Can you work these out from the model? Positions are in its coordinate system, mm. A direction names the side the tool comes from. Coordinates: 2 decimals unless noted, no trailing zeros. Order: outer loops, then holes, each group sorted by start corner. A loop starts at its lowest first (then second) coordinate and runs counter-clockwise, first axis right, second up. Notation, with made-up numbers: M 70.5,25 L 87.5,25 A31 ccw 87.5,49 Z; hole C 84.25,-21.5 d6. An arc over 180 degrees is marked long. Answer as a JSON object with one key per item and string values.
Autodesk Fusion 360 part; units mm, degrees
sketch "Sketch1" plane through (0, 0, 0) normal (1, 0, 0) x (0, 0, -1)
  circle A0 centre (-17.75, 2.25) radius 1.25
  circle A1 centre (-2.25, 2.25) radius 1.25
  circle A2 centre (-17.75, 17.75) radius 1.25
  circle A3 centre (-2.25, 17.75) radius 1.25
  circle A4 centre (-10, 10) radius 2.7
  line L0 (-13.1, 0) -> (-13.1, 1.7)
  line L1 (-13.1, 1.7) -> (-15.5, 1.7)
  line L2 (-15.5, 1.7) -> (-15.5, 3.2272)
  line L3 (-13.1, 0) -> (-20, 0)
  line L4 (-13.1, 0) -> (-6.9, 0) construction
  line L5 (-10, 15.8164) -> (-10, 4.0346) construction
  line L6 (-15.4081, 10) -> (-4.6511, 10) construction
  line L7 (-16.7728, 4.5) -> (-18.3, 4.5)
  line L8 (-18.3, 4.5) -> (-18.3, 6.9)
  line L9 (-18.3, 6.9) -> (-20, 6.9)
  line L10 (-20, 6.9) -> (-20, 0)
  line L11 (0, 6.9) -> (0, 0)
  line L12 (-1.7, 6.9) -> (0, 6.9)
  line L13 (-1.7, 4.5) -> (-1.7, 6.9)
  line L14 (-3.2272, 4.5) -> (-1.7, 4.5)
  line L15 (-4.5, 1.7) -> (-4.5, 3.2272)
  line L16 (-6.9, 1.7) -> (-4.5, 1.7)
  line L17 (-6.9, 0) -> (-6.9, 1.7)
  line L18 (-6.9, 0) -> (0, 0)
  line L19 (-6.9, 20) -> (-6.9, 18.3)
  line L20 (-6.9, 18.3) -> (-4.5, 18.3)
  line L21 (-4.5, 18.3) -> (-4.5, 16.7728)
  line L22 (-3.2272, 15.5) -> (-1.7, 15.5)
  line L23 (-1.7, 15.5) -> (-1.7, 13.1)
  line L24 (-1.7, 13.1) -> (0, 13.1)
  line L25 (0, 13.1) -> (0, 20)
  line L26 (-6.9, 20) -> (0, 20)
  line L27 (-13.1, 20) -> (-13.1, 18.3)
  line L28 (-13.1, 20) -> (-20, 20)
  line L29 (-13.1, 18.3) -> (-15.5, 18.3)
  line L30 (-15.5, 18.3) -> (-15.5, 16.7728)
  line L31 (-16.7728, 15.5) -> (-18.3, 15.5)
  line L32 (-18.3, 15.5) -> (-18.3, 13.1)
  line L33 (-18.3, 13.1) -> (-20, 13.1)
  line L34 (-20, 13.1) -> (-20, 20)
  line L35 (-16.7728, 4.5) -> (-13.8, 7.4728)
  line L36 (-7.4728, 13.8) -> (-4.5, 16.7728)
  line L37 (-15.5, 16.7728) -> (-12.5272, 13.8)
  line L38 (-6.2, 7.4728) -> (-3.2272, 4.5)
  line L39 (-15.5, 3.2272) -> (-12.5272, 6.2)
  line L40 (-6.2, 12.5272) -> (-3.2272, 15.5)
  line L41 (-16.7728, 15.5) -> (-13.8, 12.5272)
  line L42 (-7.4728, 6.2) -> (-4.5, 3.2272)
  line L43 (-12.5272, 13.8) -> (-7.4728, 13.8)
  line L44 (-6.2, 12.5272) -> (-6.2, 7.4728)
  line L45 (-7.4728, 6.2) -> (-12.5272, 6.2)
  line L46 (-13.8, 7.4728) -> (-13.8, 12.5272)
  line L47 (-17.75, 17.75) -> (-2.25, 2.25) construction
  line L48 (-17.75, 2.25) -> (-2.25, 17.75) construction
  dimension "d3" = 2.5
  dimension "d13" = 15.5
  dimension "d14" = 5.4
  dimension "d16" = 2.4
  dimension "d19" = 1.7
  dimension "d21" = 3.1
  dimension "d29" = 4.5
  dimension "d30" = 1.7
  dimension "d31" = 2.4
  dimension "d32" = 4.5
extrude "Extrude1" add sketch "Sketch1" along normal blind 300
Item 1: I want a section at A-A, the plane y = 10. Write out the boundary of the cut face in (x, z).
Answers follow:
{"outline": "M 0,6.2 L 300,6.2 L 300,7.3 L 0,7.3 Z; M 0,12.7 L 300,12.7 L 300,13.8 L 0,13.8 Z"}
Item 2: Which directions (+Z, -Z, +X, -X, +Y, -Y) give clear straight access to the entire face, cutting with the end or side of a thin tool? Please do faces 4 (the flat face through (148, 3, 0)), 5 (the flat face through (148, 13.8, 10)), 6 (the flat face through (148, 0, 3)), 7 (the flat face through (148, 10, 13.8)), 8 (the flat face through (148, 6.2, 10)).
Answers follow:
{"face 4": "-Z, +X, -X, +Y, -Y", "face 5": "+X, -X, +Y", "face 6": "+Z, -Z, +X, -X, -Y", "face 7": "+Z, +X, -X", "face 8": "+X, -X, -Y"}
Item 3: Please list where these lines run through material, in increasing order: line 1 (Y direction, x = 141, z = 17.75); line 2 (Y direction, x = 110, z = 10); line 3 (Y direction, x = 37.5, z = 18.5).
Answers follow:
{"line 1": "y = 0 to 1, 3.5 to 4.5, 15.5 to 16.5, 19 to 20", "line 2": "y = 6.2 to 7.3, 12.7 to 13.8", "line 3": "y = 0 to 1.25, 3.25 to 6.9, 13.1 to 16.75, 18.75 to 20"}
Item 4: I'm going to push flat-ended pins straight in: pin 1 (2.5 mm diameter, centred on x = 141.5, z = 9.5, fed in from -Y); pin 2 (1 mm diameter, centred on x = 150, y = 11.5, fed in from -Z). Where does each tip first touch, or does it pass through?
Answers follow:
{"pin 1": "stops at y = 6.2", "pin 2": "stops at z = 6.2"}
Item 5: I want a section at B-B, the plane x = 213.5. Give the number of separate pieces and of enclosed holes in the cut face, plus the area to 3 significant figures.
Answers follow:
{"separate pieces": "1", "enclosed holes": "5", "area": "153 mm^2"}
Item 6: If we mould it in two halves opening along Y, with no side actions, what happens to faces 1 (the flat face through (148, 10, 6.2)), 2 (the flat face through (148, 0, 17)), 3 (the flat face through (148, 17, 20))? For each: pulls with the +Y half, pulls with the -Y half, needs draft (parallel to the pull), parting line crosses it, or undercut.
Answers follow:
{"face 1": "undercut", "face 2": "pulls with the -Y half", "face 3": "needs draft"}
